```python
from build123d import *

# Parameters (mm, degrees)
BOSS_EXTRUDE1_DEPTH = 500
SKETCH2_W           = 350
SKETCH2_H           = 300
CUT_EXTRUDE1_DEPTH  = 100


with BuildPart() as part:
    # Sketch1 → Boss-Extrude1 (new body)
    with BuildSketch(Plane.XY):
        with BuildLine():
            Line((0, 0), (0, 310))
            Line((0, 310), (-3.629297392, 310))
            ThreePointArc((-3.629297392, 310), (-9.002293475, 308.433914458), (-12.692375262, 304.226182617))
            Line((-12.692375262, 304.226182617), (-147.921596127, 14.226182617))
            ThreePointArc((-147.921596127, 14.226182617), (-147.292432715, 4.627003917), (-138.858518257, 0))
            Line((-138.858518257, 0), (0, 0))
        make_face()
    extrude(amount=BOSS_EXTRUDE1_DEPTH)

    # Sketch2 → Cut-Extrude1 (cut, along a direction that is not the sketch's normal)
    with BuildSketch(Plane(origin=(-126.950826732, 59.198142714, 0), x_dir=(0, 0, 1), z_dir=(-0.906307787, 0.422618262, 0))):
        with Locations((250, 110.368730506)):
            Rectangle(SKETCH2_W, SKETCH2_H)
    extrude(amount=-CUT_EXTRUDE1_DEPTH, dir=(-1, 0, 0), mode=Mode.SUBTRACT)


solid = part.part
```
The model under review builds one solid part; all positions refer to its coordinate system, in mm. A direction names the side the tool comes from. Round coordinates to 2 decimals unless told otherwise and drop trailing zeros. Loops run counter-clockwise (first coordinate to the right, second up) from the corner with the lowest first, then second, coordinate; pieces in that order, holes last. Notation, with made-up numbers: M 17.25,-21 L 48.25,-21 A23 cw 48.25,-9 Z; hole C 37,19 d9. An arc over 180 degrees is marked long. Answer as a JSON object with one key per item and string values.
(1) Take a section at C-C on z = 55.5. Give the boundary of the cut face in (x, y).
Resolved:
{"outline": "M -147.92,14.23 A10 ccw -138.86,0 L 0,0 L 0,310 L -3.63,310 A10 ccw -12.69,304.23 Z"}
(2) Tool access review of faces 1 (the flat face through (-48, 146, 75)), 2 (the flat face through (-9, 295.172, 248)), 3 (the flat face through (-59, 123, 500)): name each direction out of +Z, -Z, +X, -X, +Y, -Y from which nothing blocks a thin tool from reaching the whole face with its end or side.
Resolved:
{"face 1": "-X", "face 2": "+X, -X", "face 3": "+Z, +X, -X, +Y, -Y"}
(3) Clearance check with a flat-ended pin moving along its axis: P1, Ø5, axis at x = -63, z = 426, coming from the +Y side. State where the tip first meets the part, or that it passes through.
Resolved:
{"P1": "y = 201.7"}
(4) Draft analysis for pull direction Y (two halves, no side actions). For faces 4 (the flat face through (-94, 23.28, 248)), 5 (the flat face through (-48, 146, 425)), 6 (the cylindrical face through (-147.37, 4.75, 246.5)), state which applies: released by +Y, released by -Y, zero draft, split by the parting line, or undercut.
Resolved:
{"face 4": "released by +Y", "face 5": "undercut", "face 6": "split by the parting line"}
(5) Take a section at A-A on y = 245. Give the boundary of the cut face in (x, z), and give its area (3 significant figures).
Resolved:
{"outline": "M -40.31,0 L 0,0 L 0,75 L -40.31,75 Z; M -40.31,425 L 0,425 L 0,500 L -40.31,500 Z", "area": "6,050 mm²"}
(6) To check wall thickness, follow line 1 along Z through (x, y) = (-114.5, 84.5); line 2 along Y through (x, z) = (-7.5, 117.5); line 3 along Y through (x, z) = (-10, 301.5). State the ranges of each line that lie inside material, in increasing order.
Resolved:
{"line 1": "0 to 75, 425 to 500", "line 2": "0 to 100.91, 295.17 to 309.22", "line 3": "0 to 95.55, 295.17 to 307.71"}
(7) Take a section at B-B on z = 250. Give the boundary of the cut face in (x, y).
Resolved:
{"outline": "M -147.92,14.23 A10 ccw -138.86,0 L 0,0 L 0,116.99 L -43.7,23.28 L -143.7,23.28 Z; M -16.91,295.17 L 0,295.17 L 0,310 L -3.63,310 A10 ccw -12.69,304.23 Z"}
(8) Take a section at D-D on x = -130.5. Give the boundary of the cut face in (y, z), and give its area (3 significant figures).
Resolved:
{"outline": "M 0,0 L 51.59,0 L 51.59,75 L 23.28,75 L 23.28,425 L 51.59,425 L 51.59,500 L 0,500 Z", "area": "15,900 mm²"}
